```python
from build123d import *

# Parameters (mm, degrees)
BOSS_EXTRUDE2_DEPTH = 1
BOSS_EXTRUDE3_DEPTH = 3


with BuildPart() as part:
    # Sketch3 → Boss-Extrude2 (new body)
    with BuildSketch(Plane(origin=(0, 0, 0), x_dir=(1, 0, 0), z_dir=(0, 1, 0))):
        Polygon((-9.140125584, 3.822331346), (1.841778899, 10.300006386), (8.641571626, 6.373357215), (8.640464915, -6.376642737), (1.901698314, -10.266239118), (-9.140125584, -3.891239118), align=None)
    extrude(amount=BOSS_EXTRUDE2_DEPTH)

    # Sketch5 → Boss-Extrude3 (add)
    with BuildSketch(Plane.XZ):
        Polygon((-9.140125584, 3.891239118), (1.901698314, 10.266239118), (2.551217367, 9.89133862), (-9.140125584, 3.14133862), align=None)
        Polygon((-9.140125584, -3.822331346), (-9.140125584, -3.06825184), (2.48777328, -9.926966588), (1.841778899, -10.300006386), align=None)
        Polygon((8.640464915, 6.376642737), (8.641571626, -6.373357215), (7.99206405, -6.748425762), (7.990892239, 6.751574187), align=None)
    extrude(amount=BOSS_EXTRUDE3_DEPTH)


solid = part.part
```
Source: CAD feature listing. Evaluate the final solid. Frame: model axes, mm. A direction names the side the tool comes from. Give positions to 0.01 mm unless a question says otherwise; leave off trailing zeros. Order: outer loops, then holes, each group sorted by start corner. A loop starts at its lowest first (then second) coordinate and runs counter-clockwise, first axis right, second up. Notation, with made-up numbers: (41, 49) -> (61, 49) arc R26 ccw to (61, 78) -> close; hole circle Ø10 at (25, -26.75). An arc over 180 degrees is marked (long way). Use a Markdown table: item, result.
Q1. Section A-A (y = -2.3). Return the cut outline in (x, z), and give its area (3 significant figures).
A:
| item | result |
|---|---|
| outline | (-9.14, -3.82) -> (1.84, -10.3) -> (2.49, -9.93) -> (-9.14, -3.07) -> close; (-9.14, 3.14) -> (2.55, 9.89) -> (1.9, 10.27) -> (-9.14, 3.89) -> close; (7.99, -6.75) -> (8.64, -6.37) -> (8.64, 6.38) -> (7.99, 6.75) -> close |
| area | 25.6 mm^2 |
Q2. Section C-C (z = 9). Return the cut outline in (x, y), and give its area (3 significant figures).
A:
| item | result |
|---|---|
| outline | (-0.29, -3) -> (1.01, -3) -> (1.01, 0) -> (4.1, 0) -> (4.1, 1) -> (-0.29, 1) -> close |
| area | 8.28 mm^2 |
Q3. Section B-B (x = 1.5). Return the cut outline in (y, z), and give its area (3 significant figures).
A:
| item | result |
|---|---|
| outline | (-3, -10.1) -> (1, -10.1) -> (1, 10.03) -> (-3, 10.03) -> (-3, 9.28) -> (0, 9.28) -> (0, -9.34) -> (-3, -9.34) -> close |
| area | 24.6 mm^2 |
Q4. Access query for faces 1 (the face through (-3.213, -1.479, 6.564)), 2 (the face through (-3.726, -1.028, -7.016)). Directions: +Z, -Z, +X, -X, +Y, -Y. A direction counts if a zero-diameter tool reaches every point of the face in a straight line with its end or side. Return the directions, or none.
A:
| item | result |
|---|---|
| face 1 | -Y |
| face 2 | -Z, -X, +Y, -Y |
Q5. Pull-direction query (X, two-part tool) for faces 3 (the face through (1, 0, 0)), 4 (the face through (-9.14, 0.4, 0)), 5 (the face through (-3, -3, -7)); classes: +X half, -X half, draft (parallel to the pull), parting line (faces both ways), or undercut.
A:
| item | result |
|---|---|
| face 3 | undercut |
| face 4 | -X half |
| face 5 | draft |
Q6. First-contact query: P1, Ø2, axis at x = -1.5, y = 0.5, coming from the +Z side; P2, Ø1, axis at x = 6, z = 6.5, coming from the -Y side. Flat tips, straight axial feed; report the tip coordinate or a pass-through.
A:
| item | result |
|---|---|
| P1 | z = 8.88 |
| P2 | y = 0 |
Q7. Section D-D (x = -6.25). Return the cut outline in (y, z).
A:
| item | result |
|---|---|
| outline | (-3, -5.53) -> (1, -5.53) -> (1, 5.56) -> (-3, 5.56) -> (-3, 4.81) -> (0, 4.81) -> (0, -4.77) -> (-3, -4.77) -> close |
Q8. Material intervals for line 1 (Y direction, x = 1.5, z = -3.5); line 2 (Z direction, x = -1.25, y = -0.6); line 3 (Z direction, x = -2.25, y = -2.7), sorted ascending. Write a range as [from, to].
A:
| item | result |
|---|---|
| line 1 | [0, 1] |
| line 2 | [-8.48, -7.72], [7.7, 8.45] |
| line 3 | [-7.89, -7.13], [7.12, 7.87] |
